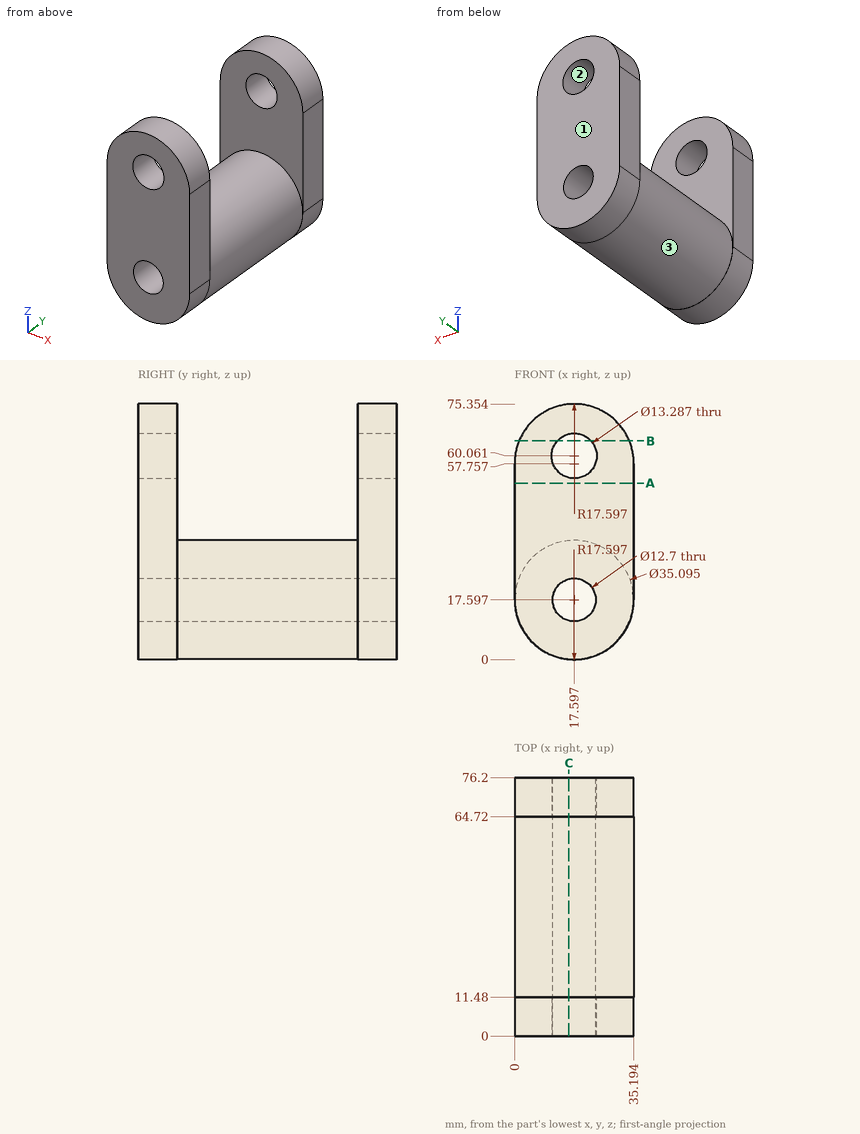
Could you check a few things on this drawing? It's one solid part, dimensions in mm from its lowest x, y, z. Round coordinates to 2 decimals unless told otherwise and drop trailing zeros. Loops run counter-clockwise (first coordinate to the right, second up) from the corner with the lowest first, then second, coordinate; pieces in that order, holes last.
Q1. Thinking about a two-plate mould opening in X: for the marked faces 1, 2 and 3, which applies, pulls with the +X half, pulls with the -X half, needs draft (parallel to the pull), parting line crosses it, or undercut?
Q2. I want a section at A-A (z = 52). Write out the boundary of the cut face in (x, y).
Q3. Please list where these lines run through material, in increasing order: L1, parallel to Y at x = 8.5, z = 47; L2, parallel to Z at x = 18, y = 59; L3, parallel to X at y = 22, z = 19.5 (1 decimal).
Q4. I want a section at C-C (x = 16). Write out the boundary of the cut face in (y, z).
Q5. For P1, Ø8, axis at x = 17.6, z = 60.06, coming from the -Y side; P2, Ø3, axis at x = 14.5, y = 28, coming from the +Z side; P3, Ø1.5, axis at x = 7.5, y = 33, coming from the -Z side (1 decimal); P4, Ø8, axis at x = 8, y = 36.5, coming from the +Z side, each with a flat end and sliding along its axis, tell me the tip position at first contact or that it passes through.
Q6. I want a section at B-B (z = 64.5). Write out the boundary of the cut face in (x, y).
Answer below:
1. face 1: needs draft
1. face 2: undercut
1. face 3: parting line crosses it
2. outline: (0, 0) - (35.19, 0) - (35.19, 11.48) - (0, 11.48) - close; (0, 64.72) - (35.19, 64.72) - (35.19, 76.2) - (0, 76.2) - close
3. L1: y = 0 to 11.48, 64.72 to 76.2
3. L2: z = 0.05 to 11.26, 23.93 to 35.14
3. L3: x = 0.2 to 11.5, 23.7 to 35
4. outline: (0, 0.07) - (11.48, 0.07) - (11.48, 0.12) - (64.72, 0.12) - (64.72, 0.07) - (76.2, 0.07) - (76.2, 11.45) - (0, 11.45) - close; (0, 23.74) - (76.2, 23.74) - (76.2, 53.61) - (64.72, 53.61) - (64.72, 35.07) - (11.48, 35.07) - (11.48, 53.61) - (0, 53.61) - close; (0, 66.51) - (11.48, 66.51) - (11.48, 75.28) - (0, 75.28) - close; (64.72, 66.51) - (76.2, 66.51) - (76.2, 75.28) - (64.72, 75.28) - close
5. P1: passes through
5. P2: stops at z = 35.07
5. P3: stops at z = 2.7
5. P4: stops at z = 34.23
6. outline: (1.34, 0) - (12.65, 0) - (12.65, 11.48) - (1.34, 11.48) - close; (1.34, 64.72) - (12.65, 64.72) - (12.65, 76.2) - (1.34, 76.2) - close; (22.54, 0) - (33.85, 0) - (33.85, 11.48) - (22.54, 11.48) - close; (22.54, 64.72) - (33.85, 64.72) - (33.85, 76.2) - (22.54, 76.2) - close
